Verification items for the finished model (mm, model axes). A direction names the side the tool comes from. Coordinates: 2 decimals unless noted, no trailing zeros. Order: outer loops, then holes, each group sorted by start corner. A loop starts at its lowest first (then second) coordinate and runs counter-clockwise, first axis right, second up. Notation, with made-up numbers: (16, 75) -> (36, 75) arc R16 ccw to (36, 83) -> close; hole circle Ø5 at (36, 38.25). An arc over 180 degrees is marked (long way). Write item = value, one per line. Start each with the question number.
1. Thickness scan on line 1 along Y through (x, z) = (-42.5, 7.5); line 2 along Y through (x, z) = (-47.5, 7.5); line 3 along Y through (x, z) = (-48.25, 7.5). Record the ranges inside material, lowest first. Write a range as from..to.
2. Cross-section at B-B on x = -50. Record the cut outline in (y, z).
3. Set-up check for faces 4 (the flat face through (-52, 320, 7)), 5 (the flat face through (-46, 395.507, 7)), 6 (the flat face through (-61, 375.507, 7)), 7 (the flat face through (-50.75, 337.72, 10.56)), 8 (the flat face through (-46.084, 306.493, 13.986)): record each of +Z, -Z, +X, -X, +Y, -Y from which the full face is reachable in a straight line by a thin tool's end or side.
4. Cross-section at A-A on z = 7.5. Record the cut outline in (x, y).
5. Cross-section at D-D on y = 384. Record the cut outline in (x, z).
6. Go/stop test with flat-tipped pins: P1, Ø2, axis at x = -48, y = 351.5, coming from the -Z side; P2, Ø4.5, axis at x = -61, z = 8.5, coming from the -Y side. Record where each tip stops, or that it passes through.
7. Release check for a two-part mould opening along X. For faces 1 (the flat face through (-42, 351, 15)), 2 (the flat face through (-43.3, 350, 11)), 3 (the flat face through (-52, 381, 7)) record: +X half, -X half, draft (parallel to the pull), parting line (faces both ways), or undercut.
8. Cross-section at C-C on x = -63.5. Record the cut outline in (y, z), plus the area to 3 significant figures.
from build123d import *

# Parameters (mm, degrees)
SKETCH_1_R          = 11.25
EXTRUDE_1_DEPTH     = 15
CHAMFER_1_SIZE      = 10
SKETCH_2_R          = 4.25
CUT_EXTRUDE_1_DEPTH = 397.745051815
CUT_EXTRUDE_2_DEPTH = 9
CHAMFER_2_SIZE      = 2


with BuildPart() as part:
    # 草图1 → 凸台-拉伸1 (new body)
    with BuildSketch(Plane.XY):
        Polygon((-52, 375.506526422), (-79.499521759, 375.506526422), (-79.499521759, 325.506526422), (-52, 325.506526422), (-52, 305.506526422), (-40, 305.506526422), (-40, 395.506526422), (-52, 395.506526422), align=None)
        with Locations((-58, 350.506526422)):
            Circle(SKETCH_1_R, mode=Mode.SUBTRACT)
    extrude(amount=EXTRUDE_1_DEPTH)

    # 倒角1
    chamfer_1_edges = [part.edges().sort_by_distance(p)[0] for p in [
        (-79.499521759, 375.506526422, 7.5),
        (-79.499521759, 325.506526422, 7.5),
    ]]
    chamfer(chamfer_1_edges, length=CHAMFER_1_SIZE)

    # 草图2 → 切除-拉伸1 (cut, through all)
    with BuildSketch(Plane.ZY.offset(52)):
        with Locations((7.5, 385.506526422)):
            Circle(SKETCH_2_R)
        with Locations((7.5, 315.506526422)):
            Circle(SKETCH_2_R)
    extrude(amount=-CUT_EXTRUDE_1_DEPTH, mode=Mode.SUBTRACT)

    # 草图3 → 切除-拉伸2 (cut)
    with BuildSketch(Plane.XY.offset(15)):
        Polygon((-58, 367.480624336), (-72.7, 358.993575379), (-72.7, 342.019477465), (-58, 333.532428508), (-43.3, 342.019477465), (-43.3, 358.993575379), align=None)
    extrude(amount=-CUT_EXTRUDE_2_DEPTH, mode=Mode.SUBTRACT)

    # 倒角2
    chamfer_2_edges = [part.edges().sort_by_distance(p)[0] for p in [
        (-46, 305.506526422, 15),
        (-46, 395.506526422, 15),
        (-46, 395.506526422, 0),
        (-46, 305.506526422, 0),
    ]]
    chamfer(chamfer_2_edges, length=CHAMFER_2_SIZE)


solid = part.part
Worked out:
q1.line_1 = 305.51..311.26, 319.76..381.26, 389.76..395.51
q1.line_2 = 305.51..311.26, 319.76..339.59, 361.42..381.26, 389.76..395.51
q1.line_3 = 305.51..311.26, 319.76..339.16, 361.85..381.26, 389.76..395.51
q2.outline = (305.51, 2) -> (307.51, 0) -> (342.6, 0) -> (342.6, 6) -> (338.15, 6) -> (338.15, 15) -> (307.51, 15) -> (305.51, 13) -> close; (358.42, 0) -> (393.51, 0) -> (395.51, 2) -> (395.51, 13) -> (393.51, 15) -> (362.86, 15) -> (362.86, 6) -> (358.42, 6) -> close; hole circle Ø8.5 at (315.51, 7.5); hole circle Ø8.5 at (385.51, 7.5)
q3.face_4 = +Z, -Z, -X, -Y
q3.face_5 = +Z, -Z, +X, -X, +Y
q3.face_6 = +Z, -Z, -X, +Y
q3.face_7 = +Z
q3.face_8 = +Z, +X, -X, -Y
q4.outline = (-79.5, 335.51) -> (-69.5, 325.51) -> (-52, 325.51) -> (-52, 319.76) -> (-40, 319.76) -> (-40, 381.26) -> (-52, 381.26) -> (-52, 375.51) -> (-69.5, 375.51) -> (-79.5, 365.51) -> close; (-52, 305.51) -> (-40, 305.51) -> (-40, 311.26) -> (-52, 311.26) -> close; (-52, 389.76) -> (-40, 389.76) -> (-40, 395.51) -> (-52, 395.51) -> close; hole (-72.7, 342.02) -> (-58, 333.53) -> (-43.3, 342.02) -> (-43.3, 358.99) -> (-58, 367.48) -> (-72.7, 358.99) -> close
q5.outline = (-52, 0) -> (-40, 0) -> (-40, 3.53) -> (-52, 3.53) -> close; (-52, 11.47) -> (-40, 11.47) -> (-40, 15) -> (-52, 15) -> close
q6.P1 = through
q6.P2 = 325.51
q7.face_1 = draft
q7.face_2 = undercut
q7.face_3 = -X half
q8.outline = (325.51, 0) -> (340.69, 0) -> (340.69, 6) -> (336.71, 6) -> (336.71, 15) -> (325.51, 15) -> close; (360.32, 0) -> (375.51, 0) -> (375.51, 15) -> (364.31, 15) -> (364.31, 6) -> (360.32, 6) -> close
q8.area = 384 mm²
